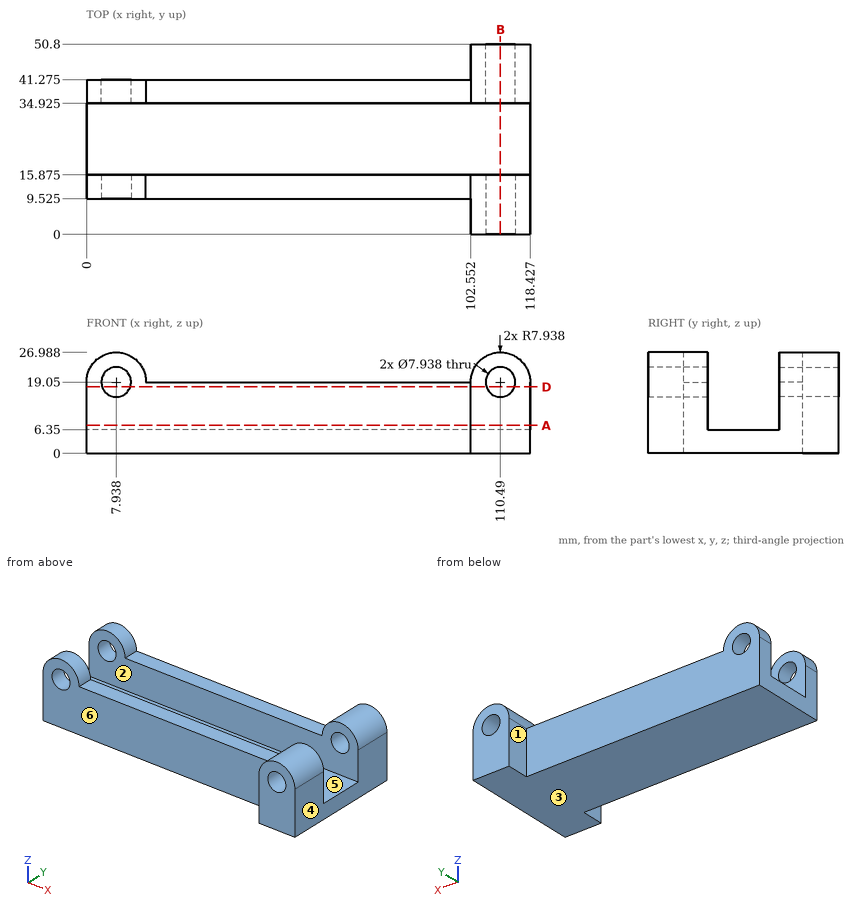
Part print with two shaded views. Sizes in mm from the minimum x, y, z corner. A direction names the side the tool comes from. Give positions to 0.01 mm unless a question says otherwise; leave off trailing zeros. Order: outer loops, then holes, each group sorted by start corner. A loop starts at its lowest first (then second) coordinate and runs counter-clockwise, first axis right, second up.
1) 3-axis set-ups, long thin cutter, end or side, ignore diameter. For the marked faces 1, 2 and 3: which of +Z, -Z, +X, -X, +Y, -Y reach the whole face in a straight line?
2) Wall check: probe 1 along Y at (x, z) = (79, 12) (1 decimal); probe 2 along Y at (x, z) = (103.5, 11) (1 decimal); probe 3 along X at (y, z) = (40, 18) (1 decimal). Give the ranges that are in metal, low to high.
3) Saw through at B-B, the plane x = 110.49. Count the separate pieces of the cut face and the enclosed holes in it, then the cut area to 3 significant figures.
4) Saw through at A-A, the plane z = 7.5. Write the cut outline in (x, y) (1 decimal), then the cut area to 3 significant figures.
5) Pin check, flat tips, straight feed: pin 1 (7 mm diameter, centred on x = 75, y = 14, fed in from +Z); pin 2 (8 mm diameter, centred on x = 41, z = 12.5, fed in from -Y) (1 decimal); pin 3 (3 mm diameter, centred on y = 5, z = 10.5, fed in from -X); pin 4 (8 mm diameter, centred on x = 61.5, z = 23.5, fed in from +Y). Stop position of each tip, or through.
6) Saw through at D-D, the plane z = 17.75. Write the cut outline in (x, y) (1 decimal).
7) Mould opens along Y. For the marked faces 4, 5 and 6 say: +Y half, -Y half, draft (parallel to the pull), parting line (faces both ways), or undercut.
Computed:
1. face 1: +Z, -Z, -X, +Y
1. face 2: +Z, +X, -X
1. face 3: -Z, +X, -X, +Y, -Y
2. probe 1: y = 9.5 to 15.9, 34.9 to 41.3
2. probe 2: y = 0 to 15.9, 34.9 to 50.8
2. probe 3: x = 0 to 4.1, 11.8 to 106.7, 114.3 to 118.4
3. separate pieces: 3
3. enclosed holes: 0
3. area: 726 mm2
4. outline: (0, 9.5) - (102.6, 9.5) - (102.6, 0) - (118.4, 0) - (118.4, 15.9) - (0, 15.9) - close; (0, 34.9) - (118.4, 34.9) - (118.4, 50.8) - (102.6, 50.8) - (102.6, 41.3) - (0, 41.3) - close
4. area: 1,810 mm2
5. pin 1: stops at z = 19.05
5. pin 2: stops at y = 9.5
5. pin 3: stops at x = 102.55
5. pin 4: passes through
6. outline: (0, 9.5) - (4.2, 9.5) - (4.2, 15.9) - (0, 15.9) - close; (0, 34.9) - (4.2, 34.9) - (4.2, 41.3) - (0, 41.3) - close; (11.7, 9.5) - (102.6, 9.5) - (102.6, 0) - (106.7, 0) - (106.7, 15.9) - (11.7, 15.9) - close; (11.7, 34.9) - (106.7, 34.9) - (106.7, 50.8) - (102.6, 50.8) - (102.6, 41.3) - (11.7, 41.3) - close; (114.2, 0) - (118.4, 0) - (118.4, 15.9) - (114.2, 15.9) - close; (114.2, 34.9) - (118.4, 34.9) - (118.4, 50.8) - (114.2, 50.8) - close
7. face 4: draft
7. face 5: undercut
7. face 6: -Y half
